Here's how the part is built. I have some questions about the finished solid (model axes, mm). Face numbers are marked on the shaded views. A direction names the side the tool comes from. Round coordinates to 2 decimals unless told otherwise and drop trailing zeros. Write each loop counter-clockwise with the first axis right and the second up, starting at its lowest first coordinate (ties: lowest second). Pieces come first, ordered by that corner, then holes. Notation, with made-up numbers: (-29, 2) - (-25, 2) arc R27 cw to (-25, 32) - close; hole circle Ø3 at (-7.75, 48). An arc over 180 degrees is marked (long way). One line per question, with ' | ' between items. Start each with the question number.
(1) If I drill on L1, parallel to X at y = 2, z = 7.5; L2, parallel to X at y = 2.75, z = 7; L3, parallel to Y at x = -9.5, z = -3.5, over which ranges is the centre line in solid material (lowest first)?
(2) Will these pins go through, and if not, where does the flat tip stop? pin 1 (3 mm diameter, centred on x = -14, z = -2, fed in from -Y); pin 2 (2 mm diameter, centred on x = 0, z = 8, fed in from -Y); pin 3 (13 mm diameter, centred on x = -6, z = -10.5, fed in from +Y); pin 4 (5 mm diameter, centred on x = -16.5, z = -8, fed in from +Y).
(3) Imagine slicing it at B-B (x = -12). Write out the boundary of the cut face in (y, z), plus the area to 3 significant figures.
(4) Imagine slicing it at A-A (z = 16). Write out the boundary of the cut face in (x, y), plus the area to 3 significant figures.
(5) Imagine slicing it at D-D (y = 5). Write out the boundary of the cut face in (x, z).
(6) Thinking about a two-plate mould opening in X: for the marked faces 4, 5 and 6, which applies, pulls with the +X half, pulls with the -X half, needs draft (parallel to the pull), parting line crosses it, or undercut?
(7) Imagine slicing it at C-C (y = 2.5). Write out the boundary of the cut face in (x, z).
(8) For the marked faces 1, 2 and 3, which set-ups out of +Z, -Z, +X, -X, +Y, -Y let a thin tool reach every point of the face, with its end or its side?
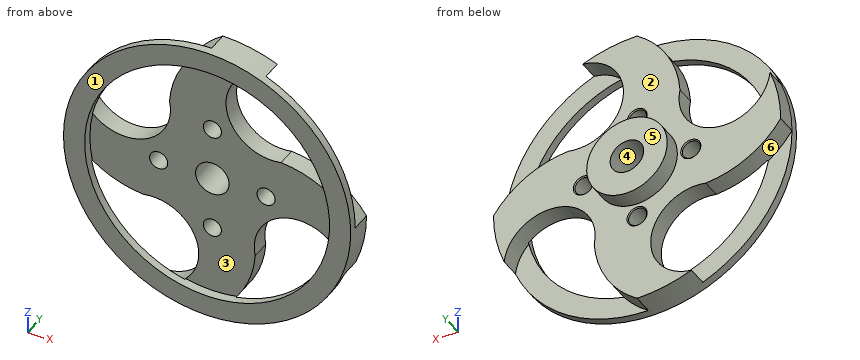
from build123d import *

# Parameters (mm, degrees)
SKETCH_4_R                = 21.4
EXTRUDE_2_DEPTH           = 1.2
EXTRUDE_5_DEPTH           = 4.2
SKETCH_7_R                = 18.25
CUT_EXTRUDE_2_DEPTH       = 1.4
SKETCH_9_R                = 6
EXTRUDE_6_DEPTH           = 2.7
SKETCH_10_R               = 2.5
CUT_EXTRUDE_3_DEPTH       = 32.040779629
HOLE_WIZARD_1_D           = 2.7
HOLE_WIZARD_1_CSINK_D     = 3
HOLE_WIZARD_1_CSINK_ANGLE = 90


with BuildPart() as part:
    # 草图4 → 凸台-拉伸2 (new body)
    with BuildSketch(Plane(origin=(0, 0, 0), x_dir=(1, 0, 0), z_dir=(0, 1, 0))):
        with Locations(Location((0, 0, 0), (0, 0, 270))):
            Circle(SKETCH_4_R)
    extrude(amount=EXTRUDE_2_DEPTH)

    # 草图5 → 凸台-拉伸5 (add)
    with BuildSketch(Plane(origin=(0, 0, 0), x_dir=(1, 0, 0), z_dir=(0, 1, 0))):
        with BuildLine():
            ThreePointArc((0, 21.4), (-4.129005127, 20.997888386), (-8.102840074, 19.806665109))
            ThreePointArc((-8.102840074, 19.806665109), (-2.113798114, 11.981054753), (-10.229363001, 6.391206133))
            ThreePointArc((-10.229363001, 6.391206133), (-16.561312382, 4.500574676), (-21.4, 0))
            ThreePointArc((-21.4, 0), (-20.997888386, -4.129005127), (-19.806665109, -8.102840074))
            ThreePointArc((-19.806665109, -8.102840074), (-11.981054753, -2.113798114), (-6.391206133, -10.229363001))
            ThreePointArc((-6.391206133, -10.229363001), (-4.500574676, -16.561312382), (0, -21.4))
            ThreePointArc((0, -21.4), (4.129005127, -20.997888386), (8.102840074, -19.806665109))
            ThreePointArc((8.102840074, -19.806665109), (2.113798114, -11.981054753), (10.229363001, -6.391206133))
            ThreePointArc((10.229363001, -6.391206133), (16.561312382, -4.500574676), (21.4, 0))
            ThreePointArc((21.4, 0), (20.997888386, 4.129005127), (19.806665109, 8.102840074))
            ThreePointArc((19.806665109, 8.102840074), (11.981054753, 2.113798114), (6.391206133, 10.229363001))
            ThreePointArc((6.391206133, 10.229363001), (4.500574676, 16.561312382), (0, 21.4))
        make_face()
    extrude(amount=EXTRUDE_5_DEPTH)

    # 草图7 → 切除-拉伸2 (cut)
    with BuildSketch(Plane.XZ):
        with Locations(Location((0, 0, 0), (0, 0, 270))):
            Circle(SKETCH_7_R)
    extrude(amount=-CUT_EXTRUDE_2_DEPTH, mode=Mode.SUBTRACT)

    # 草图9 → 凸台-拉伸6 (add)
    with BuildSketch(Plane(origin=(0, 4.2, 0), x_dir=(1, 0, 0), z_dir=(0, 1, 0))):
        with Locations(Location((0, 0, 0), (0, 0, 90))):
            Circle(SKETCH_9_R)
    extrude(amount=EXTRUDE_6_DEPTH)

    # 草图10 → 切除-拉伸3 (cut, through all)
    with BuildSketch(Plane(origin=(0, 6.9, 0), x_dir=(1, 0, 0), z_dir=(0, 1, 0))):
        with Locations(Location((0, 0, 0), (0, 0, 270))):
            Circle(SKETCH_10_R)
    extrude(amount=-CUT_EXTRUDE_3_DEPTH, mode=Mode.SUBTRACT)

    # 打孔尺寸(%根据)内六角花形半沉头螺钉的类型1 (through all)
    with Locations(Plane(origin=(-8, 4.2, 0), x_dir=(0, 0, 1), z_dir=(0, 1, 0))):
        with Locations((0, 0), (-8, 8), (0, 16), (8, 8)):
            CounterSinkHole(HOLE_WIZARD_1_D / 2, HOLE_WIZARD_1_CSINK_D / 2, counter_sink_angle=HOLE_WIZARD_1_CSINK_ANGLE)


solid = part.part
Check sheet entries:
1) L1: -20.04 to -19.71, -6.38 to -1.25, 1.25 to 4.89 | L2: -20.22 to -19.59, -6.5 to -0.91, 0.91 to 5.72 | L3: 1.4 to 4.2
2) pin 1: y = 1.4 | pin 2: through | pin 3: y = 6.9 | pin 4: y = 1.2
3) outline: (0, -17.72) - (1.2, -17.72) - (1.2, -13.75) - (0, -13.75) - close; (0, 13.75) - (1.2, 13.75) - (1.2, 17.72) - (0, 17.72) - close; (1.4, -6.17) - (4.2, -6.17) - (4.2, 2.11) - (1.4, 2.11) - close | area: 32.7 mm^2
4) outline: (-14.21, 0) - (-8.78, 0) - (-8.78, 1.2) - (-14.21, 1.2) - close; (-4.81, 1.4) - (2.71, 1.4) - (2.71, 4.2) - (-4.81, 4.2) - close; (8.78, 0) - (14.21, 0) - (14.21, 1.2) - (8.78, 1.2) - close | area: 34.1 mm^2
5) outline: circle Ø12 at (0, 0); hole circle Ø5 at (0, 0)
6) face 4: undercut | face 5: needs draft | face 6: pulls with the -X half
7) outline: (-21.4, 0) arc R14.52 ccw to (-10.23, -6.39) arc R6.8 cw (long way) to (-8.1, -19.81) arc R21.4 ccw to (0, -21.4) arc R14.52 ccw to (6.39, -10.23) arc R6.8 cw (long way) to (19.81, -8.1) arc R21.4 ccw to (21.4, 0) arc R14.52 ccw to (10.23, 6.39) arc R6.8 cw (long way) to (8.1, 19.81) arc R21.4 ccw to (0, 21.4) arc R14.52 ccw to (-6.39, 10.23) arc R6.8 cw (long way) to (-19.81, 8.1) arc R21.4 ccw to start; hole circle Ø2.7 at (-8, 0); hole circle Ø5 at (0, 0); hole circle Ø2.7 at (0, -8); hole circle Ø2.7 at (0, 8); hole circle Ø2.7 at (8, 0)
8) face 1: +Z, -Z, +X, -X, -Y | face 2: +Y | face 3: -Y
